Build history of the part. All positions in model axes, mm. Face numbers are marked on the shaded views. A direction names the side the tool comes from. Round coordinates to 2 decimals unless told otherwise and drop trailing zeros. Write each loop counter-clockwise with the first axis right and the second up, starting at its lowest first coordinate (ties: lowest second). Pieces come first, ordered by that corner, then holes. Notation, with made-up numbers: (22, 30) -> (59, 30) arc R12 ccw to (59, 52) -> close; hole circle Ø7 at (23, 81). An arc over 180 degrees is marked (long way). Return JSON: item names as keys, results as strings.
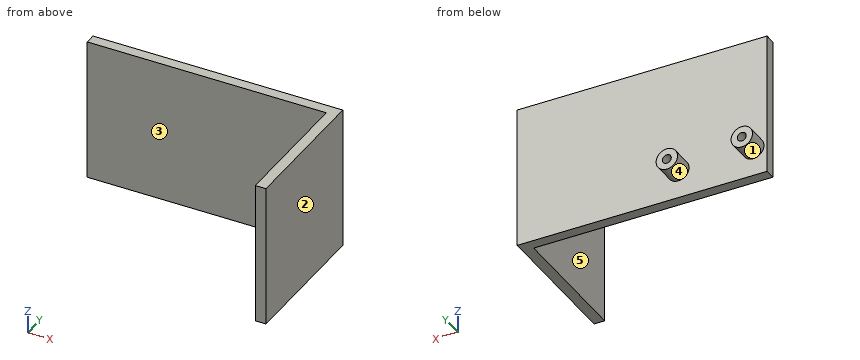
from build123d import *

# Parameters (mm, degrees)
SKETCH1_W                       = 70
SKETCH1_H                       = 40
BOSS_EXTRUDE1_DEPTH             = 40
SKETCH2_W                       = 40
SKETCH2_H                       = 37
CUT_EXTRUDE1_DEPTH              = 67
SKETCH4_R                       = 3
BOSS_EXTRUDE2_DEPTH             = 6
TAP_DRILL_FOR_M3X0_5_TAP2_D     = 2.5
TAP_DRILL_FOR_M3X0_5_TAP2_DEPTH = 6
TAP_DRILL_FOR_M3X0_5_TAP2_TIP   = 0.751075774


with BuildPart() as part:
    # Sketch1 → Boss-Extrude1 (new body)
    with BuildSketch(Plane(origin=(0, 0, 0), x_dir=(1, 0, 0), z_dir=(0, 1, 0))):
        Rectangle(SKETCH1_W, SKETCH1_H)
    extrude(amount=BOSS_EXTRUDE1_DEPTH)

    # Sketch2 → Cut-Extrude1 (cut)
    with BuildSketch(Plane.ZY.offset(35)):
        with Locations((0, 18.5)):
            Rectangle(SKETCH2_W, SKETCH2_H)
    extrude(amount=-CUT_EXTRUDE1_DEPTH, mode=Mode.SUBTRACT)

    # Sketch4 → Boss-Extrude2 (add)
    with BuildSketch(Plane(origin=(0, 40, 0), x_dir=(1, 0, 0), z_dir=(0, 1, 0))):
        with Locations((-31.149822544, 12.062768)):
            Circle(SKETCH4_R)
        with Locations((-10.149822544, 12.062768)):
            Circle(SKETCH4_R)
    extrude(amount=BOSS_EXTRUDE2_DEPTH)

    # Tap Drill for M3x0.5 Tap2
    with Locations(Plane(origin=(0, 46, 0), x_dir=(1, 0, 0), z_dir=(0, 1, 0))):
        with Locations((-31.149822544, 12.062768), (-10.149822544, 12.062768)):
            Hole(TAP_DRILL_FOR_M3X0_5_TAP2_D / 2, depth=TAP_DRILL_FOR_M3X0_5_TAP2_DEPTH)
            with Locations((0, 0, -(TAP_DRILL_FOR_M3X0_5_TAP2_DEPTH + TAP_DRILL_FOR_M3X0_5_TAP2_TIP / 2))):  # 118° drill point
                Cone(0, TAP_DRILL_FOR_M3X0_5_TAP2_D / 2, TAP_DRILL_FOR_M3X0_5_TAP2_TIP, mode=Mode.SUBTRACT)


solid = part.part
Q1. 3-axis set-ups, long thin cutter, end or side, ignore diameter. For the marked faces 4 and 5: which of +Z, -Z, +X, -X, +Y, -Y reach the whole face in a straight line?
Verdict:
{"face 4": "+Y", "face 5": "+Z, -Z, -X, -Y"}
Q2. Saw through at C-C on x = 15.5. List the corners of the cut face in (y, z), then the cut area to 3 significant figures.
Verdict:
{"outline": "(37, -20) -> (40, -20) -> (40, 20) -> (37, 20) -> close", "area": "120 mm²"}
Q3. Saw through at A-A on z = 16.5. List the corners of the cut face in (x, y).
Verdict:
{"outline": "(-35, 37) -> (32, 37) -> (32, 0) -> (35, 0) -> (35, 40) -> (-35, 40) -> close"}
Q4. Two-plate mould, pull along X, no slides. Class the marked faces 1, 2 and 3: +X half, -X half, draft (parallel to the pull), parting line (faces both ways), or undercut.
Verdict:
{"face 1": "undercut", "face 2": "+X half", "face 3": "draft"}
Q5. Wall check: L1, parallel to Y at x = 7.5, z = -2; L2, parallel to X at y = 12, z = -7. Give the ranges that are in metal, low to high.
Verdict:
{"L1": "y = 37 to 40", "L2": "x = 32 to 35"}
Q6. Pin check, flat tips, straight feed: pin 1 Ø1 at (x, y) = (-4, 35.5) entering from -Z; pin 2 Ø10 at (x, z) = (26.5, 11) entering from +Y; pin 3 Ø3 at (x, z) = (-31.15, -12.06) entering from +Y; pin 4 Ø1.5 at (y, z) = (23.5, 12.5) entering from -X. Stop position of each tip, or through.
Verdict:
{"pin 1": "passes through", "pin 2": "stops at y = 40", "pin 3": "stops at y = 46", "pin 4": "stops at x = 32"}
Q7. Saw through at B-B on y = 31. List the corners of the cut face in (x, z), then the cut area to 3 significant figures.
Verdict:
{"outline": "(32, -20) -> (35, -20) -> (35, 20) -> (32, 20) -> close", "area": "120 mm²"}
Q8. Saw through at D-D on z = -10. List the corners of the cut face in (x, y).
Verdict:
{"outline": "(-35, 37) -> (32, 37) -> (32, 0) -> (35, 0) -> (35, 40) -> (-7.97, 40) -> (-7.97, 46) -> (-12.33, 46) -> (-12.33, 40) -> (-28.97, 40) -> (-28.97, 46) -> (-33.33, 46) -> (-33.33, 40) -> (-35, 40) -> close"}
